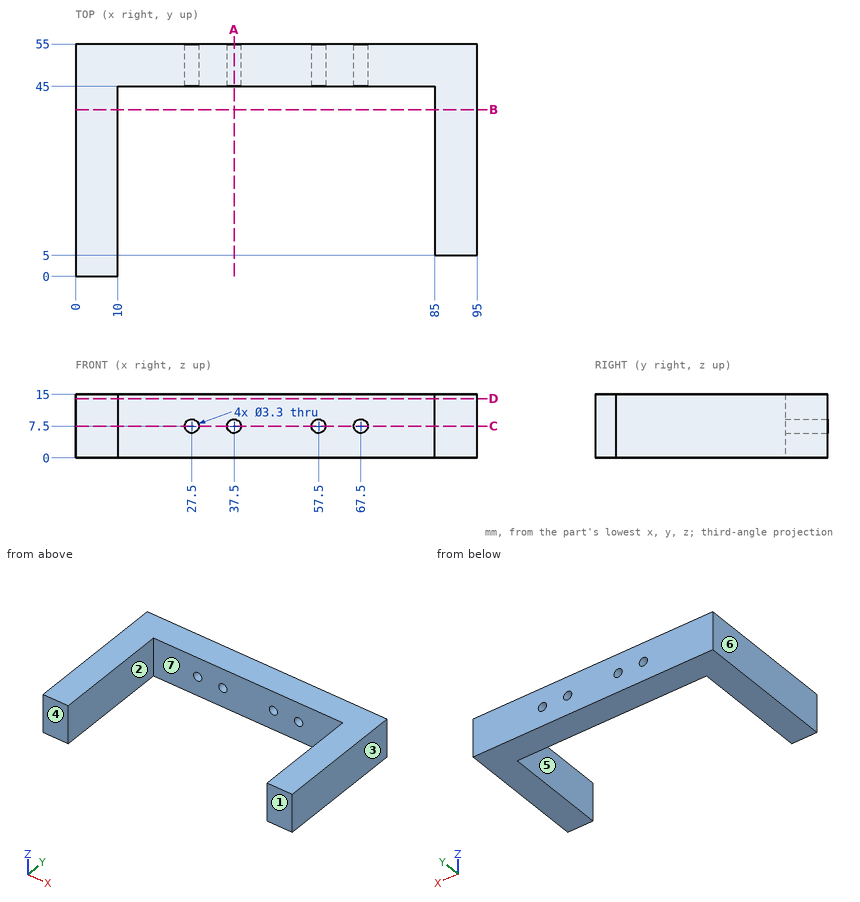
Study the drawing (mm; zero at the part's minimum x, y, z) and answer. A direction names the side the tool comes from. Round coordinates to 2 decimals unless told otherwise and drop trailing zeros. Write each loop counter-clockwise with the first axis right and the second up, starting at its lowest first coordinate (ties: lowest second). Pieces come first, ordered by that corner, then holes.
1) A tool of negligible diameter and unlimited length cuts with its end or side. For the marked faces 1, 2 and 3, from which of +Z, -Z, +X, -X, +Y, -Y can it reach the whole face along a straight path? Write none if from no direction.
2) The mould has two halves that part along X. Classify the marked faces 4, 5, 6 and 7: pulls with the +X half, pulls with the -X half, needs draft (parallel to the pull), parting line crosses it, or undercut.
3) Straight lines are drawn through the part: line 1 (X direction, y = 47.5, z = 7.5); line 2 (Z direction, x = 37.5, y = 50.75); line 3 (X direction, y = 34.5, z = 3.5). For each, find the intervals that lie inside material, in ascending order.
4) A cutting plane is placed at D-D (z = 14). Give the vertices of the cut face in (x, y), plus the area to 3 significant figures.
5) A cutting plane is placed at A-A (x = 37.5). Give the vertices of the cut face in (y, z).
6) A cutting plane is placed at C-C (z = 7.5). Give the vertices of the cut face in (x, y).
7) A cutting plane is placed at B-B (y = 39.5). Give the vertices of the cut face in (x, z), plus the area to 3 significant figures.
8) Given pin 1 Ø5 at (x, z) = (90, 10) entering from -Y; pin 2 Ø4 at (x, z) = (37.5, 7.5) entering from -Y, each flat-ended and moving along its own axis, determine where each tip first touches the part or whether it passes through.
Completed:
1. face 1: +Z, -Z, +X, -Y
1. face 2: +Z, -Z, -Y
1. face 3: +Z, -Z, +X, +Y, -Y
2. face 4: needs draft
2. face 5: undercut
2. face 6: pulls with the -X half
2. face 7: undercut
3. line 1: x = 0 to 25.85, 29.15 to 35.85, 39.15 to 55.85, 59.15 to 65.85, 69.15 to 95
3. line 2: z = 0 to 5.85, 9.15 to 15
3. line 3: x = 0 to 10, 85 to 95
4. outline: (0, 0) - (10, 0) - (10, 45) - (85, 45) - (85, 5) - (95, 5) - (95, 55) - (0, 55) - close
4. area: 1,800 mm2
5. outline: (45, 0) - (55, 0) - (55, 5.85) - (45, 5.85) - close; (45, 9.15) - (55, 9.15) - (55, 15) - (45, 15) - close
6. outline: (0, 0) - (10, 0) - (10, 45) - (25.85, 45) - (25.85, 55) - (0, 55) - close; (29.15, 45) - (35.85, 45) - (35.85, 55) - (29.15, 55) - close; (39.15, 45) - (55.85, 45) - (55.85, 55) - (39.15, 55) - close; (59.15, 45) - (65.85, 45) - (65.85, 55) - (59.15, 55) - close; (69.15, 45) - (85, 45) - (85, 5) - (95, 5) - (95, 55) - (69.15, 55) - close
7. outline: (0, 0) - (10, 0) - (10, 15) - (0, 15) - close; (85, 0) - (95, 0) - (95, 15) - (85, 15) - close
7. area: 300 mm2
8. pin 1: stops at y = 5
8. pin 2: stops at y = 45
